Read the model definition and answer for the solid it produces. Units are mm, in the model's axes. Face numbers are marked on the shaded views. Give positions to 0.01 mm unless a question says otherwise; leave off trailing zeros. Order: outer loops, then holes, each group sorted by start corner. A loop starts at its lowest first (then second) coordinate and runs counter-clockwise, first axis right, second up. Notation, with made-up numbers: (57, 71) - (107, 71) arc R29 ccw to (107, 109) - close; hole circle Ø11 at (9.25, -0.75). An arc over 180 degrees is marked (long way). Return JSON: item names as keys, results as strings.
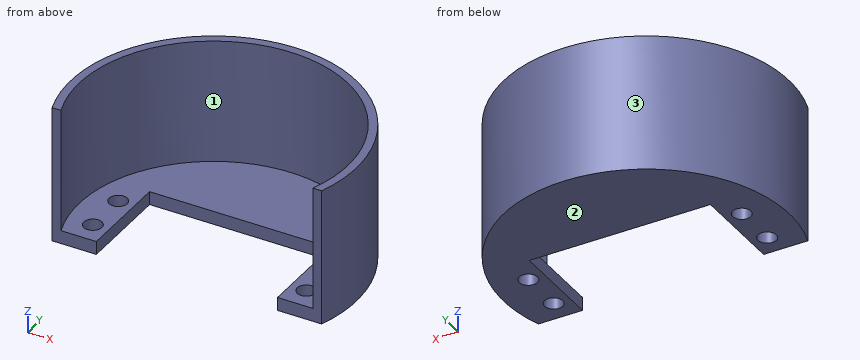
```python
from build123d import *

# Parameters (mm, degrees)
CROQUIS1_R              = 2.060946668
SALIENTE_EXTRUIR1_DEPTH = 3
SALIENTE_EXTRUIR2_DEPTH = 28


with BuildPart() as part:
    # Croquis1 → Saliente-Extruir1 (new body)
    with BuildSketch(Plane.XY):
        with BuildLine():
            Line((-17.644764035, 22.151573595), (23.355235965, 22.151573595))
            Line((23.355235965, 22.151573595), (23.355235965, 1.151573595))
            Line((23.355235965, 1.151573595), (33.355235965, 1.151573595))
            ThreePointArc((33.355235965, 1.151573595), (2.855235965, 43.908355827), (-27.644764035, 1.151573595))
            Line((-27.644764035, 1.151573595), (-17.644764035, 1.151573595))
            Line((-17.644764035, 1.151573595), (-17.644764035, 22.151573595))
        make_face()
        with Locations((27.005235965, 6.151573595)):
            Circle(CROQUIS1_R, mode=Mode.SUBTRACT)
        with Locations((-21.294764035, 6.151573595)):
            Circle(CROQUIS1_R, mode=Mode.SUBTRACT)
        with Locations((-21.294764035, 16.151573595)):
            Circle(CROQUIS1_R, mode=Mode.SUBTRACT)
        with Locations((27.005235965, 16.151573595)):
            Circle(CROQUIS1_R, mode=Mode.SUBTRACT)
    extrude(amount=SALIENTE_EXTRUIR1_DEPTH)

    # Croquis2 → Saliente-Extruir2 (add)
    with BuildSketch(Plane.XY.offset(3)):
        with BuildLine():
            Line((-27.644764035, 1.151573595), (-25.644764035, 1.151573595))
            ThreePointArc((-25.644764035, 1.151573595), (2.855235965, 42.024258692), (31.355235965, 1.151573595))
            Line((31.355235965, 1.151573595), (33.355235965, 1.151573595))
            ThreePointArc((33.355235965, 1.151573595), (2.855235965, 43.908355827), (-27.644764035, 1.151573595))
        make_face()
    extrude(amount=SALIENTE_EXTRUIR2_DEPTH)


solid = part.part
```
Q1. A cutting plane is placed at D-D (z = 18). Write down the section's boundary in (x, y).
Values:
{"outline": "(-27.64, 1.15) - (-25.64, 1.15) arc R30.37 cw (long way) to (31.36, 1.15) - (33.36, 1.15) arc R32.26 ccw (long way) to start"}
Q2. A cutting plane is placed at B-B (x = -18.5). Write down the section's boundary in (y, z), and give its area (3 significant figures).
Values:
{"outline": "(1.15, 0) - (35.83, 0) - (35.83, 31) - (33.25, 31) - (33.25, 3) - (1.15, 3) - close", "area": "176 mm²"}
Q3. Consider L1, parallel to X at y = 12, z = 13; L2, parallel to Z at x = 7.5, y = 36; L3, parallel to X at y = 36, z = 8.5. Determine where each line is inside the solid, lowest interval first.
Values:
{"L1": "x = -29.4 to -27.52, 33.23 to 35.11", "L2": "z = 0 to 3", "L3": "x = -18.3 to -15.3, 21.01 to 24.01"}
Q4. A cutting plane is placed at A-A (y = 10). Write down the section's boundary in (x, z), and give its area (3 significant figures).
Values:
{"outline": "(-29.36, 0) - (-17.64, 0) - (-17.64, 3) - (-27.47, 3) - (-27.47, 31) - (-29.36, 31) - close; (23.36, 0) - (35.07, 0) - (35.07, 31) - (33.18, 31) - (33.18, 3) - (23.36, 3) - close", "area": "176 mm²"}
Q5. Given pin 1 (12 mm diameter, centred on x = 20, z = 18.5, fed in from -Y); pin 2 (6 mm diameter, centred on y = 18, z = 17.5, fed in from +X); pin 3 (5.5 mm diameter, centred on x = -21.29, y = 6.15, fed in from -Z); pin 4 (10 mm diameter, centred on y = 32, z = 25.5, fed in from -X), each flat-ended and moving along its own axis, determine where each tip first touches the part or whether it passes through.
Values:
{"pin 1": "stops at y = 31.32", "pin 2": "stops at x = 34.94", "pin 3": "stops at z = 0", "pin 4": "stops at x = -25.52"}
Q6. A cutting plane is placed at C-C (y = 21). Write down the section's boundary in (x, z), and give its area (3 significant figures).
Values:
{"outline": "(-28.02, 0) - (-17.64, 0) - (-17.64, 3) - (-26.04, 3) - (-26.04, 31) - (-28.02, 31) - close; (23.36, 0) - (33.73, 0) - (33.73, 31) - (31.75, 31) - (31.75, 3) - (23.36, 3) - close", "area": "173 mm²"}
Q7. Determine the mould class of the marked faces 1, 2 and 3 for opening direction Y: released by +Y, released by -Y, zero draft, split by the parting line, or undercut.
Values:
{"face 1": "undercut", "face 2": "zero draft", "face 3": "split by the parting line"}
